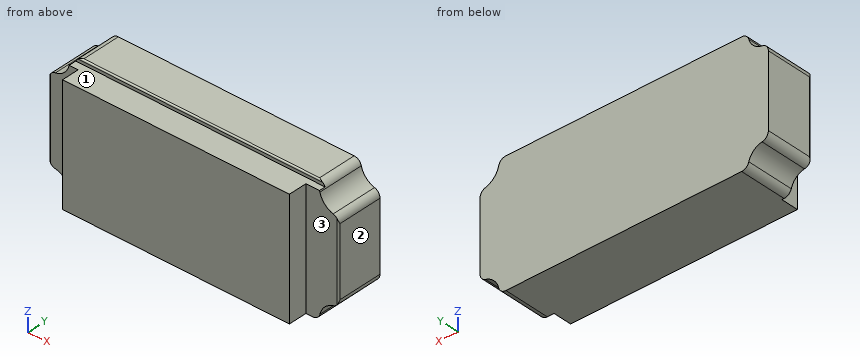
from build123d import *
from OCP.BRepAlgoAPI import BRepAlgoAPI_Cut
from OCP.TopTools import TopTools_ListOfShape

# Parameters (mm, degrees)
BOSS_EXTRUDE1_DEPTH     = 21.85
CUT_EXTRUDE1_DEPTH      = 48.4
CUT_EXTRUDE1_DEPTH_BACK = 48.4
CUT_EXTRUDE2_DEPTH      = 20.5
CUT_EXTRUDE2_DEPTH_BACK = 20.5


with BuildPart() as part:
    # Sketch1 → Boss-Extrude1 (new body)
    with BuildSketch(Plane(origin=(0, 0, 0), x_dir=(1, 0, 0), z_dir=(0, 1, 0))):
        with BuildLine():
            Line((-48.4, 12.151203914), (-48.4, -12.151203914))
            ThreePointArc((-48.4, -12.151203914), (-47.79906628, -13.773402604), (-46.286322418, -14.612602183))
            ThreePointArc((-46.286322418, -14.612602183), (-43.456956945, -15.955525197), (-41.833947517, -18.63406801))
            ThreePointArc((-41.833947517, -18.63406801), (-40.94758788, -19.979013629), (-39.423420787, -20.5))
            Line((-39.423420787, -20.5), (39.709565228, -20.5))
            ThreePointArc((39.709565228, -20.5), (41.256886583, -19.960870735), (42.134162778, -18.57694508))
            ThreePointArc((42.134162778, -18.57694508), (43.717900388, -15.664841516), (46.568112128, -13.972250299))
            ThreePointArc((46.568112128, -13.972250299), (47.889747358, -13.080993613), (48.4, -11.570794818))
            Line((48.4, -11.570794818), (48.4, 11.570794818))
            ThreePointArc((48.4, 11.570794818), (47.889747358, 13.080993613), (46.568112128, 13.972250299))
            ThreePointArc((46.568112128, 13.972250299), (43.717900388, 15.664841516), (42.134162778, 18.57694508))
            ThreePointArc((42.134162778, 18.57694508), (41.256886583, 19.960870735), (39.709565228, 20.5))
            Line((39.709565228, 20.5), (-39.423420787, 20.5))
            ThreePointArc((-39.423420787, 20.5), (-40.94758788, 19.979013629), (-41.833947517, 18.63406801))
            ThreePointArc((-41.833947517, 18.63406801), (-43.456956895, 15.955525241), (-46.286322286, 14.612602203))
            ThreePointArc((-46.286322286, 14.612602203), (-47.799066237, 13.773402654), (-48.4, 12.151203914))
        make_face()
    extrude(amount=BOSS_EXTRUDE1_DEPTH)

    # Sketch2 → Cut-Extrude1 (cut, two sides: drawn at the far end of the back side and taken through both)
    with BuildSketch(Plane(origin=(0, 0, 0), x_dir=(0, 0, -1), z_dir=(1, 0, 0)).offset(-CUT_EXTRUDE1_DEPTH_BACK)):
        with BuildLine():
            Line((-20.5, 8.85), (-20.5, 0))
            Line((-20.5, 0), (-19, 0))
            Line((-19, 0), (-19, 8.35))
            Line((-19, 8.35), (-20, 8.35))
            ThreePointArc((-20, 8.35), (-20.353553391, 8.496446609), (-20.5, 8.85))
        make_face()
    extrude(amount=CUT_EXTRUDE1_DEPTH + CUT_EXTRUDE1_DEPTH_BACK, mode=Mode.SUBTRACT)


with BuildPart() as cut_extrude2_tool:
    # Sketch3 → Cut-Extrude2 (new, two sides: drawn at the far end of the back side and taken through both)
    with BuildSketch(Plane.XY.offset(-CUT_EXTRUDE2_DEPTH_BACK)):
        with BuildLine():
            Line((-48.4, -5), (48.4, -5))
            Line((48.4, -5), (48.4, 6.75))
            ThreePointArc((48.4, 6.75), (48.253553391, 6.396446609), (47.9, 6.25))
            Line((47.9, 6.25), (37.44, 6.25))
            Line((37.44, 6.25), (37.44, 0))
            Line((37.44, 0), (-38.7, 0))
            Line((-38.7, 0), (-38.7, 5.85))
            Line((-38.7, 5.85), (-47.9, 5.85))
            ThreePointArc((-47.9, 5.85), (-48.253553391, 5.996446609), (-48.4, 6.35))
            Line((-48.4, 6.35), (-48.4, -5))
        make_face()
    extrude(amount=CUT_EXTRUDE2_DEPTH + CUT_EXTRUDE2_DEPTH_BACK)


with BuildPart() as part_1:
    add(part.part)

    # Cut-Extrude2: cut by cut_extrude2_tool, with a tolerance
    cut_extrude2_stock = TopTools_ListOfShape()
    cut_extrude2_stock.Append(part_1.part.wrapped)
    cut_extrude2_tools = TopTools_ListOfShape()
    cut_extrude2_tools.Append(cut_extrude2_tool.part.wrapped)
    cut_extrude2_cut = BRepAlgoAPI_Cut()
    cut_extrude2_cut.SetArguments(cut_extrude2_stock)
    cut_extrude2_cut.SetTools(cut_extrude2_tools)
    cut_extrude2_cut.SetFuzzyValue(0.00001)
    cut_extrude2_cut.Build()
    add(Compound.cast(cut_extrude2_cut.Shape()).solids(), mode=Mode.REPLACE)


solid = part_1.part
For this review, take the finished solid that the model builds, in its own axes (mm). Face numbers are marked on the shaded views. A direction names the side the tool comes from. Coordinates: 2 decimals unless noted, no trailing zeros. Loops run counter-clockwise (first coordinate to the right, second up) from the corner with the lowest first, then second, coordinate; pieces in that order, holes last. Notation, with made-up numbers: (58, -39.75) - (74, -39.75) arc R20 cw to (74, -1.75) - close; hole circle Ø10 at (43, 88). An arc over 180 degrees is marked (long way). Use a Markdown table: item, result. Add a question column.
Item 1: Tool access review of the marked faces 1, 2 and 3: name each direction out of +Z, -Z, +X, -X, +Y, -Y from which nothing blocks a thin tool from reaching the whole face with its end or side.
Item 2: Insertion check: pin 1 Ø3 at (x, y) = (11.5, 5.5) entering from +Z; pin 2 Ø8.5 at (x, z) = (42, -8.5) entering from -Y; pin 3 Ø1.9 at (y, z) = (3, -7) entering from +X. Each pin has a flat end and moves straight along its axis. Give the tip position at first contact, or say it passes through.
Item 3: We need section A-A (x = 38.5). Give the boundary of the cut face in (y, z), and give its area (3 significant figures).
Item 4: We need section C-C (z = -17). Give the boundary of the cut face in (x, y), and give its area (3 significant figures).
Item 5: For line 1 (Z direction, x = -38, y = 6.5); line 2 (Y direction, x = -43, z = -14.5); line 3 (X direction, y = 1.75, z = -11), list the stretches that pass through material, from the lowest coordinate up.
Item 6: We need section B-B (z = -8.5). Give the boundary of the cut face in (x, y), and give its area (3 significant figures).
Results list:
| question | item | result |
|---|---|---|
| 1 | face 1 | +Z, +X, -X, -Y |
| 1 | face 2 | +Z, -Z, +X, +Y, -Y |
| 1 | face 3 | +Z, -Z, +X, -Y |
| 2 | pin 1 | stops at z = 19 |
| 2 | pin 2 | stops at y = 6.25 |
| 2 | pin 3 | stops at x = 37.44 |
| 3 | outline | (6.25, -20.5) - (21.85, -20.5) - (21.85, 20.5) - (8.85, 20.5) arc R0.5 ccw to (8.35, 20) - (8.35, 19) - (6.25, 19) - close |
| 3 | area | 636 mm^2 |
| 4 | outline | (-42.56, 5.85) - (-38.7, 5.85) - (-38.7, 0) - (37.44, 0) - (37.44, 6.25) - (42.74, 6.25) - (42.74, 21.85) - (-42.56, 21.85) - close |
| 4 | area | 1,810 mm^2 |
| 5 | line 1 | z = -20.5 to 19 |
| 5 | line 2 | y = 5.85 to 21.85 |
| 5 | line 3 | x = -38.7 to 37.44 |
| 6 | outline | (-48.4, 6.35) arc R0.5 ccw to (-47.9, 5.85) - (-38.7, 5.85) - (-38.7, 0) - (37.44, 0) - (37.44, 6.25) - (47.9, 6.25) arc R0.5 ccw to (48.4, 6.75) - (48.4, 21.85) - (-48.4, 21.85) - close |
| 6 | area | 1,990 mm^2 |
